from build123d import *

# Parameters (mm, degrees)
F0_R     = 0.5
F1_DEPTH = 62.5
F3_DEPTH = 1.5


with BuildPart() as f1:
    # F0 (on Top) → F1 (new body, symmetric)
    with BuildSketch(Plane.XY):
        Circle(F0_R)
    extrude(amount=F1_DEPTH, both=True)

    # F2 (on Right) → F3 (join, symmetric)
    with BuildSketch(Plane.YZ):
        with BuildLine():
            ThreePointArc((1.936492, 62.5), (3.44572, 63.968494), (4, 66))
            ThreePointArc((4, 66), (-2.031506, 69.44572), (-1.936492, 62.5))
            Line((-1.936492, 62.5), (1.936492, 62.5))
        make_face()
    extrude(amount=F3_DEPTH, both=True)


solid = f1.part
Build history of the part. All positions in model axes, mm. A direction names the side the tool comes from. Round coordinates to 2 decimals unless told otherwise and drop trailing zeros. Write each loop counter-clockwise with the first axis right and the second up, starting at its lowest first coordinate (ties: lowest second). Pieces come first, ordered by that corner, then holes. Notation, with made-up numbers: M 38.5,69.25 L 42.5,69.25 A20 cw 42.5,83.25 Z; hole C 50.5,-18.75 d8. An arc over 180 degrees is marked long. Answer as a JSON object with one key per item and string values. Group by question number.
(1) Cut at B-B (z = 15). Give the cut face in (x, y), and give its area (3 significant figures).
(2) Which spindle directions (+Z, -Z, +X, -X, +Y, -Y) get a long thin tool onto all of the face, cutting with end or side? Do faces 1 (the flat face through (-1, 0, 62.5)), 2 (the flat face through (1.5, 0, 66)). Say none if no direction does.
(3) Drill centre lines: L1, parallel to Z at x = -1.25, y = 0.25; L2, parallel to Y at x = 0.05, z = 51.5; L3, parallel to Z at x = 0.7, y = -3. Where is each one in solid material? Low to high.
(4) Flat gauge pin, fed straight in: pin 1 (1 mm diameter, centred on x = 0, z = -45, fed in from -Y). Where does the tip first touch, or does it go through?
(5) Cut at A-A (x = 0). Give the cut face in (y, z), and give its area (3 significant figures).
Responses:
{
 "1": {"outline": "C 0,0 d1", "area": "0.785 mm2"},
 "2": {"face 1": "-Z", "face 2": "+Z, -Z, +X, +Y, -Y"},
 "3": {"L1": "z = 62.5 to 69.99", "L2": "y = -0.5 to 0.5", "L3": "z = 63.35 to 68.65"},
 "4": {"pin 1": "stops at y = -0.5"},
 "5": {"outline": "M -1.94,62.5 L -0.5,62.5 L -0.5,-62.5 L 0.5,-62.5 L 0.5,62.5 L 1.94,62.5 A4 ccw 4,66 A4 ccw long Z", "area": "174 mm2"}
}
